Study the drawing (mm; zero at the part's minimum x, y, z) and answer. A direction names the side the tool comes from. Round coordinates to 2 decimals unless told otherwise and drop trailing zeros. Write each loop counter-clockwise with the first axis right and the second up, starting at its lowest first coordinate (ties: lowest second). Pieces come first, ordered by that corner, then holes. Notation, with made-up numbers: M 32,-7.75 L 67,-7.75 A17 ccw 67,1.25 Z; hole C 69.5,61 d2. An arc over 180 degrees is marked long. Write each question's results on one line, items separated by ' | '.
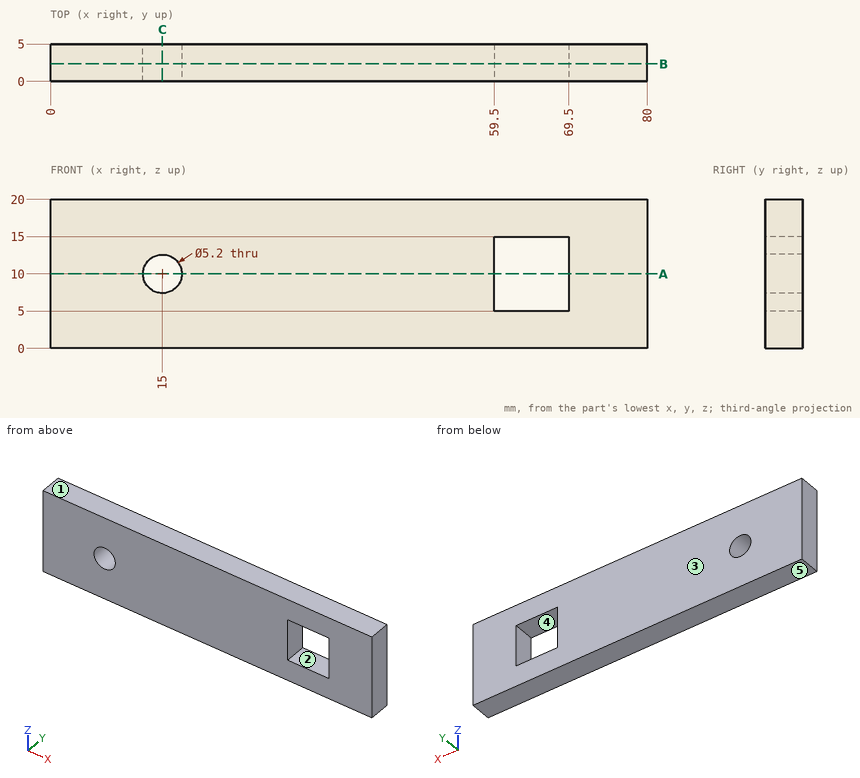
1) Section A-A (z = 10) is taken. Determine the outline of the cut face in (x, y).
Return value:
outline: M 0,0 L 12.4,0 L 12.4,5 L 0,5 Z; M 17.6,0 L 59.5,0 L 59.5,5 L 17.6,5 Z; M 69.5,0 L 80,0 L 80,5 L 69.5,5 Z
2) This flat-tipped pin is pushed along its axis until it touches: pin 1 (3 mm diameter, centred on x = 15, z = 10, fed in from +Y). Where does it stop, or does it pass through?
Return value:
pin 1: through
3) Find the intervals of material crossed by line 1 (Z direction, x = 63.5, y = 2.8); line 2 (Z direction, x = 15, y = 2.2); line 3 (X direction, y = 3.4, z = 10.25), in increasing order.
Return value:
line 1: 0 to 5, 15 to 20 | line 2: 0 to 7.4, 12.6 to 20 | line 3: 0 to 12.41, 17.59 to 59.5, 69.5 to 80
4) Section C-C (x = 15) is taken. Determine the outline of the cut face in (y, z).
Return value:
outline: M 0,0 L 5,0 L 5,7.4 L 0,7.4 Z; M 0,12.6 L 5,12.6 L 5,20 L 0,20 Z
5) The mould has two halves that part along Z. Classify the marked faces 3, 4 and 5: +Z half, -Z half, draft (parallel to the pull), parting line (faces both ways), or undercut.
Return value:
face 3: draft | face 4: undercut | face 5: -Z half
6) Section B-B (y = 2.35) is taken. Determine the outline of the cut face in (x, z).
Return value:
outline: M 0,0 L 80,0 L 80,20 L 0,20 Z; hole C 15,10 d5.2; hole M 59.5,5 L 69.5,5 L 69.5,15 L 59.5,15 Z
7) A tool of negligible diameter and unlimited length cuts with its end or side. For the marked faces 1 and 2, from which of +Z, -Z, +X, -X, +Y, -Y can it reach the whole face along a straight path? Write none if from no direction.
Return value:
face 1: +Z, +X, -X, +Y, -Y | face 2: +Y, -Y
